Check sheet for the modelled part. Datum: model origin and axes. Units: mm. Face numbers are marked on the shaded views. A direction names the side the tool comes from. Round coordinates to 2 decimals unless told otherwise and drop trailing zeros. Order: outer loops, then holes, each group sorted by start corner. A loop starts at its lowest first (then second) coordinate and runs counter-clockwise, first axis right, second up. Notation, with made-up numbers: (-6.5, -27.5) -> (27.5, -27.5) arc R11 ccw to (27.5, -8.5) -> close; hole circle Ø8 at (71, -36). An arc over 180 degrees is marked (long way). Answer in a Markdown table with one row per item. Add a question column.
1. Sectioned sample at D-D, the plane y = 59.5. Record the boundary of the cut face in (x, z).
2. Depth check by flat-ended pin: P1, Ø3.5, axis at y = -93.5, z = -18, coming from the -X side; P2, Ø8, axis at y = 35.5, z = -40.5, coming from the -X side; P3, Ø3.5, axis at x = -42.86, y = -95, coming from the -Z side. Enter the tip coordinate at first touch or a pass-through.
3. Material ranges on L1, parallel to Y at x = 0, z = 3; L2, parallel to X at y = -48, z = -43; L3, parallel to X at y = 92, z = -46, recorded low to high. Write a range as from..to.
4. Draft check along Y on the marked faces 4, 5, 6 and 7. Enter one of: +Y half, -Y half, draft (parallel to the pull), parting line (faces both ways), or undercut.
5. Sectioned sample at B-B, the plane x = 0. Record the boundary of the cut face in (y, z), then the cut area to 3 significant figures.
6. Access from +Z, -Z, +X, -X, +Y, -Y to the whole of each face (thin tool, end or side, straight path). Record for the marked faces 1, 2 and 3.
7. Sectioned sample at A-A, the plane y = -50. Record the boundary of the cut face in (x, z), then the cut area to 4 significant figures.
8. Sectioned sample at C-C, the plane z = -44. Count the separate pieces of the cut face and the enclosed holes in it, then the cut area to 3 significant figures.
```python
from build123d import *

# Parameters (mm, degrees)
BOSS_EXTRUDE1_DEPTH     = 50
BOSS_EXTRUDE1_2_DEPTH   = 50
BOSS_EXTRUDE2_DEPTH     = 10
CHAMFER1_SIZE           = 15
CHAMFER1_SIZE_2         = 20
SKETCH4_W               = 160
SKETCH4_H               = 200
BOSS_EXTRUDE3_DEPTH     = 5
FILLET1_R               = 10
SKETCH5_R               = 7.5
CUT_EXTRUDE1_DEPTH      = 5
CUT_EXTRUDE5_DEPTH      = 140.373598648
CUT_EXTRUDE5_DEPTH_BACK = 140.373598648
FILLET4_R               = 5
SKETCH12_R              = 2
CUT_EXTRUDE6_DEPTH      = 10
SKETCH13_W              = 22.9
SKETCH13_H              = 1.9875
CUT_EXTRUDE7_DEPTH      = 50
FILLET5_R               = 1


with BuildPart() as part:
    # Sketch2 → Boss-Extrude1 (new body)
    with BuildSketch(Plane.XY):
        with BuildLine():
            Line((-50, 75), (-22.70223243, 0))
            Line((-22.70223243, 0), (-37.64392369, -17.092022104))
            ThreePointArc((-37.64392369, -17.092022104), (-49.971924127, -51.675350432), (-35.355339059, -85.355339059))
            Line((-35.355339059, -85.355339059), (-35.355339059, -100))
            Line((-35.355339059, -100), (-80, -100))
            Line((-80, -100), (-80, 100))
            Line((-80, 100), (-50, 100))
            Line((-50, 100), (-50, 75))
        make_face()
    extrude(amount=-BOSS_EXTRUDE1_DEPTH)



with BuildPart() as body_2:
    # Sketch2 → Boss-Extrude1 2 (new body)
    with BuildSketch(Plane.XY):
        with BuildLine():
            Line((50, 75), (22.70223243, 0))
            Line((22.70223243, 0), (37.64392369, -17.092022104))
            ThreePointArc((37.64392369, -17.092022104), (49.971924127, -51.675350432), (35.355339059, -85.355339059))
            Line((35.355339059, -85.355339059), (35.355339059, -100))
            Line((35.355339059, -100), (80, -100))
            Line((80, -100), (80, 100))
            Line((80, 100), (50, 100))
            Line((50, 100), (50, 75))
        make_face()
    extrude(amount=-BOSS_EXTRUDE1_2_DEPTH)


with BuildPart() as part_1:
    add(part.part)

    add(body_2.part)  # Boss-Extrude2 merges body 2
    # Sketch3 → Boss-Extrude2 (add)
    with BuildSketch(Plane.XY):
        Polygon((-29.981637115, 20), (29.981637115, 20), (22.70223243, 0), (-22.70223243, 0), align=None)
    extrude(amount=-BOSS_EXTRUDE2_DEPTH)

    # Chamfer1
    # the kernel refuses this chamfer: 20, 15 mm, written as the material it takes off along each edge
    with BuildSketch(Plane(origin=(-81.595588718, 20, -10), x_dir=(0, 0.041308380137954244, 0.9991464445867674), z_dir=(1, 0, 0))) as chamfer1_piece_1_section:
        Polygon((CHAMFER1_SIZE * 0.999146444587, CHAMFER1_SIZE * 0.041308380138), (-CHAMFER1_SIZE_2 * 0.041308380138, CHAMFER1_SIZE_2 * 0.999146444587), (0, 0), align=None)
    chamfer1_piece_1 = extrude(amount=163.191177435, mode=Mode.PRIVATE)
    chamfer1_piece_1 = split(chamfer1_piece_1, bisect_by=Plane(origin=(-24.447399798, 4.794807938, -4.975922198), z_dir=(0.9396926207859094, 0.3420201433256661, 0)), keep=Keep.TOP, mode=Mode.PRIVATE)
    chamfer1_piece_1 = split(chamfer1_piece_1, bisect_by=Plane(origin=(24.447399798, 4.794807938, -4.975922198), z_dir=(-0.939692620785907, 0.34202014332567265, 0)), keep=Keep.TOP, mode=Mode.PRIVATE)
    add(chamfer1_piece_1, mode=Mode.SUBTRACT)

    # Sketch4 → Boss-Extrude3 (add)
    with BuildSketch(Plane.XY):
        Rectangle(SKETCH4_W, SKETCH4_H)
    extrude(amount=BOSS_EXTRUDE3_DEPTH)

    # Fillet1
    fillet1_edges = [part_1.edges().sort_by_distance(p)[0] for p in [
        (-22.70223243, 0, -30),
        (-35.355339059, -85.355339059, -25),
        (35.355339059, -85.355339059, -25),
        (22.70223243, 0, -30),
        (0, 13.333333333, 0),
    ]]
    fillet(fillet1_edges, radius=FILLET1_R)

    # Sketch5 → Cut-Extrude1 (cut)
    with BuildSketch(Plane(origin=(0, 0, 0), x_dir=(-1, 0, 0), z_dir=(0, 0, -1))):
        with Locations((0, -50)):
            Circle(SKETCH5_R)
    extrude(amount=-CUT_EXTRUDE1_DEPTH, mode=Mode.SUBTRACT)

    # Sketch11 → Cut-Extrude5 (cut, two sides: drawn at the far end of the back side and taken through both)
    with BuildSketch(Plane(origin=(0, 0, -50), x_dir=(-1, 0, 0), z_dir=(0, 0, -1)).offset(-CUT_EXTRUDE5_DEPTH_BACK)):
        with BuildLine():
            Line((-58.784198233, -62.017405631), (-51.672968794, -96.802610845))
            ThreePointArc((-51.672968794, -96.802610845), (-51.161121522, -98.466118532), (-50.338653833, -100))
            Line((-50.338653833, -100), (-80, -100))
            Line((-80, -100), (-80, 100))
            Line((-80, 100), (-62.474937186, 100))
            ThreePointArc((-62.474937186, 100), (-66.199502533, 94.806221081), (-65.536970349, 88.4494312))
            Line((-65.536970349, 88.4494312), (-60, 73.236730193))
            Line((-60, 73.236730193), (-34.120235365, 2.132661237))
            Line((-34.120235365, 2.132661237), (-45.172708428, -10.510426525))
            ThreePointArc((-45.172708428, -10.510426525), (-58.008635864, -34.670350128), (-58.784198233, -62.017405631))
        make_face()
        with BuildLine():
            Line((34.120235365, 2.132661237), (45.172708428, -10.510426525))
            ThreePointArc((45.172708428, -10.510426525), (58.008635864, -34.670350128), (58.784198233, -62.017405631))
            Line((58.784198233, -62.017405631), (51.672968794, -96.802610845))
            ThreePointArc((51.672968794, -96.802610845), (51.161121522, -98.466118532), (50.338653833, -100))
            Line((50.338653833, -100), (80, -100))
            Line((80, -100), (80, 100))
            Line((80, 100), (62.474937186, 100))
            ThreePointArc((62.474937186, 100), (66.199502533, 94.806221081), (65.536970349, 88.4494312))
            Line((65.536970349, 88.4494312), (60, 73.236730193))
            Line((60, 73.236730193), (34.120235365, 2.132661237))
        make_face()
    extrude(amount=CUT_EXTRUDE5_DEPTH + CUT_EXTRUDE5_DEPTH_BACK, mode=Mode.SUBTRACT)

    # Fillet4
    fillet4_edges = [part_1.edges().sort_by_distance(p)[0] for p in [
        (-35.355339059, -100, -25),
        (-50, 100, -25),
        (62.474937186, 100, -22.5),
        (-62.474937186, 100, -22.5),
        (50, 100, -25),
        (35.355339059, -100, -25),
    ]]
    fillet(fillet4_edges, radius=FILLET4_R)

    # Sketch12 → Cut-Extrude6 (cut)
    with BuildSketch(Plane(origin=(0, 0, -50), x_dir=(-1, 0, 0), z_dir=(0, 0, -1))):
        with Locations((-57.5, 92.5)):
            Circle(SKETCH12_R)
        with Locations((57.5, 92.5)):
            Circle(SKETCH12_R)
        with Locations((-42.855339059, -95)):
            Circle(SKETCH12_R)
        with Locations((42.855339059, -95)):
            Circle(SKETCH12_R)
    extrude(amount=-CUT_EXTRUDE6_DEPTH, mode=Mode.SUBTRACT)

    # Sketch13 → Cut-Extrude7 (cut)
    with BuildSketch(Plane(origin=(0, 0, -50), x_dir=(-1, 0, 0), z_dir=(0, 0, -1))):
        with Locations((-34.105339059, -88.485929464)):
            Rectangle(SKETCH13_W, SKETCH13_H)
        with Locations((34.105339059, -88.485929464)):
            Rectangle(SKETCH13_W, SKETCH13_H)
    extrude(amount=-CUT_EXTRUDE7_DEPTH, mode=Mode.SUBTRACT)

    # Fillet5
    fillet5_edges = [part_1.edges().sort_by_distance(p)[0] for p in [
        (-35.516393803, -87.492179464, -25),
        (35.516393803, -87.492179464, -25),
        (35.355339059, -89.479679464, -25),
        (-35.355339059, -89.479679464, -25),
    ]]
    fillet(fillet5_edges, radius=FILLET5_R)


solid = part_1.part
```
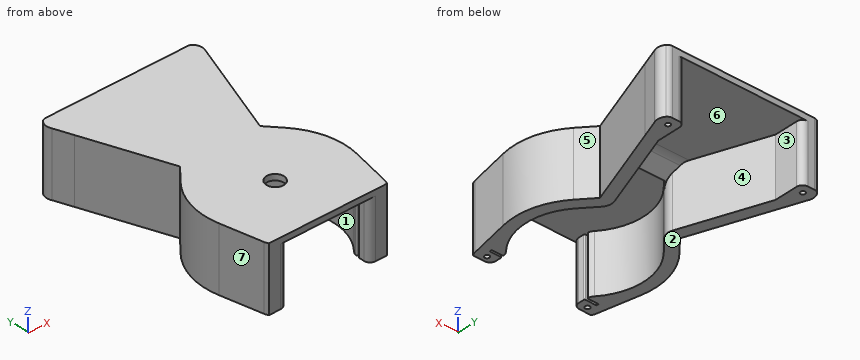
Answer key:
| question | item | result |
|---|---|---|
| 1 | outline | (-55, -50) -> (-44.36, -50) -> (-44.36, 0) -> (44.36, 0) -> (44.36, -50) -> (55, -50) -> (55, 5) -> (-55, 5) -> close |
| 2 | P1 | stops at x = -52.71 |
| 2 | P2 | stops at x = -47.72 |
| 2 | P3 | stops at z = -40 |
| 3 | L1 | y = -100..-57.5, -42.5..100 |
| 3 | L2 | x = -59.97..-49.96, 49.96..59.97 |
| 3 | L3 | x = -66.49..-59.44, -55.56..-50, 50..55.56, 59.44..66.49 |
| 4 | face 4 | +Y half |
| 4 | face 5 | undercut |
| 4 | face 6 | draft |
| 4 | face 7 | -Y half |
| 5 | outline | (-100, 0) -> (-57.5, 0) -> (-57.5, 5) -> (-100, 5) -> close; (-42.5, 0) -> (0, 0) -> (0, -10) -> (10.67, -2) arc R10 cw to (16.67, 0) -> (100, 0) -> (100, 5) -> (-42.5, 5) -> close |
| 5 | area | 993 mm² |
| 6 | face 1 | -Z |
| 6 | face 2 | -Z, +X, -X, +Y, -Y |
| 6 | face 3 | -Z, +Y |
| 7 | outline | (-60, -50) -> (-50, -50) -> (-50, 0) -> (-7.5, 0) -> (-7.5, 5) -> (-60, 5) -> close; (7.5, 0) -> (50, 0) -> (50, -50) -> (60, -50) -> (60, 5) -> (7.5, 5) -> close |
| 7 | area | 1,525 mm² |
| 8 | separate pieces | 2 |
| 8 | enclosed holes | 4 |
| 8 | area | 4,690 mm² |
